Here's how the part is built. I have some questions about the finished solid (model axes, mm). A direction names the side the tool comes from. Round coordinates to 2 decimals unless told otherwise and drop trailing zeros. Loops run counter-clockwise (first coordinate to the right, second up) from the corner with the lowest first, then second, coordinate; pieces in that order, holes last. Notation, with made-up numbers: M -19.75,11 L -13.75,11 A24 cw -13.75,45 Z; hole C -28,-31 d3. An arc over 180 degrees is marked long. Use a Markdown table: item, result.
```python
from build123d import *

# Parameters (mm, degrees)
SWEEP1_PROFILE_R    = 3
BOSS_EXTRUDE1_DEPTH = 5


with BuildPart() as part:
    # Sweep1: sweep along a path in Sketch1
    with BuildLine(Plane.XY) as sweep1_path:
        Line((-28.5, -42.5), (-28.5, 0))
        ThreePointArc((-28.5, 0), (0, 28.5), (28.5, 0))
        Line((28.5, 0), (28.5, -42.5))
    # Sweep1 profile (on start of the path) → Sweep1 (sweep)
    with BuildSketch(Plane(origin=(-28.5, -42.5, 0), x_dir=(1, 0, 0), z_dir=(0, 1, 0))):
        Circle(SWEEP1_PROFILE_R)
    sweep(path=sweep1_path.line)

    # Sketch14 → Boss-Extrude1 (add)
    with BuildSketch(Plane(origin=(0, -39, 0), x_dir=(1, 0, 0), z_dir=(0, 1, 0))):
        Polygon((-28.5, 5.773502692), (-33.5, 2.886751346), (-33.5, -2.886751346), (-28.5, -5.773502692), (-23.5, -2.886751346), (-23.5, 2.886751346), align=None)
        Polygon((23.5, 2.886751346), (28.5, 5.773502692), (33.5, 2.886751346), (33.5, -2.886751346), (28.5, -5.773502692), (23.5, -2.886751346), align=None)
    extrude(amount=-BOSS_EXTRUDE1_DEPTH)


solid = part.part
```
Q1. We'd pull the mould along X, two halves only. Please class faces 1 (the flat face through (25.965, -41.465, -4.31)), 2 (the flat face through (31.035, -41.465, 4.31)), 3 (the flat face through (29, -44, 0)): pulls with the +X half, pulls with the -X half, needs draft (parallel to the pull), parting line crosses it, or undercut.
Return value:
| item | result |
|---|---|
| face 1 | undercut |
| face 2 | pulls with the +X half |
| face 3 | needs draft |
Q2. I need wall thicknesses on line 1 (Y direction, x = 29, z = -5); line 2 (X direction, y = 5.5, z = -1.5); line 3 (X direction, y = -24, z = 0.25). Which ranges of each line are inside material? Lowest first, please. Write a range as from..to.
Return value:
| item | result |
|---|---|
| line 1 | y = -44..-39 |
| line 2 | x = -30.61..-25.31, 25.31..30.61 |
| line 3 | x = -31.49..-25.51, 25.51..31.49 |
Q3. Will these pins go through, and if not, where does the flat tip stop? P1, Ø5, axis at y = -33, z = 0, coming from the -X side; P2, Ø6, axis at x = -17.5, z = 3, coming from the -Y side; P3, Ø5, axis at x = 30.5, z = 2, coming from the +Y side.
Return value:
| item | result |
|---|---|
| P1 | stops at x = -31.5 |
| P2 | stops at y = 16.32 |
| P3 | stops at y = 13.63 |
Q4. For faces 4 (the flat face through (-23.5, -41, 0)), 5 (the flat face through (30.965, -41.465, -4.35)), 6 (the flat face through (31, -39, 2)), which set-ups out of +Z, -Z, +X, -X, +Y, -Y let a thin tool reach every point of the face, with its end or its side?
Return value:
| item | result |
|---|---|
| face 4 | +Z, -Z, -Y |
| face 5 | -Z, +X, +Y, -Y |
| face 6 | none |
Q5. Imagine slicing it at B-B, the plane y = -8. Please give me the cut outline in (x, z), then the cut area to 3 significant figures.
Return value:
| item | result |
|---|---|
| outline | C -28.5,0 d6; C 28.5,0 d6 |
| area | 56.5 mm^2 |
Q6. Imagine slicing it at C-C, the plane z = 0. Please give me the cut outline in (x, y).
Return value:
| item | result |
|---|---|
| outline | M -33.5,-44 L -23.5,-44 L -23.5,-39 L -25.5,-39 L -25.5,0 A25.5 cw 25.5,0 L 25.5,-39 L 23.5,-39 L 23.5,-44 L 33.5,-44 L 33.5,-39 L 31.5,-39 L 31.5,0 A31.5 ccw -31.5,0 L -31.5,-39 L -33.5,-39 Z |
Q7. Imagine slicing it at A-A, the plane z = -4.5. Please give me the cut outline in (x, y).
Return value:
| item | result |
|---|---|
| outline | M -30.71,-44 L -26.29,-44 L -26.29,-39 L -30.71,-39 Z; M 26.29,-44 L 30.71,-44 L 30.71,-39 L 26.29,-39 Z |
